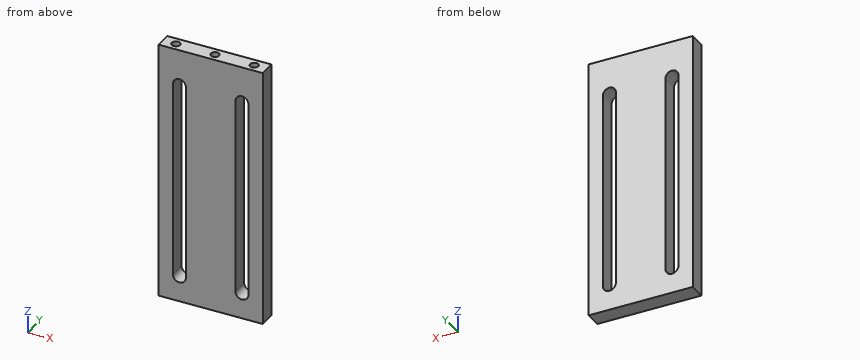
from build123d import *

# Parameters (mm, degrees)
SKETCH1_W           = 20
SKETCH1_H           = 50
BOSS_EXTRUDE1_DEPTH = 3.18
CUT_EXTRUDE1_DEPTH  = 54.94545764
SKETCH3_R           = 0.8
CUT_EXTRUDE2_DEPTH  = 4


with BuildPart() as part:
    # Sketch1 → Boss-Extrude1 (new body)
    with BuildSketch(Plane(origin=(0, 0, 0), x_dir=(1, 0, 0), z_dir=(0, 1, 0))):
        with Locations((10, 25)):
            Rectangle(SKETCH1_W, SKETCH1_H)
    extrude(amount=BOSS_EXTRUDE1_DEPTH)

    # Sketch2 → Cut-Extrude1 (cut, through all)
    with BuildSketch(Plane(origin=(0, 3.18, 0), x_dir=(1, 0, 0), z_dir=(0, 1, 0))):
        with BuildLine():
            Line((2.75, 7), (2.75, 45))
            ThreePointArc((2.75, 45), (4, 46.25), (5.25, 45))
            Line((5.25, 45), (5.25, 7))
            ThreePointArc((5.25, 7), (4, 5.75), (2.75, 7))
        make_face()
    cut_extrude1 = extrude(amount=-CUT_EXTRUDE1_DEPTH, mode=Mode.SUBTRACT)

    # Mirror1: Cut-Extrude1 across plane
    add(cut_extrude1.mirror(Plane(origin=(10, 0, 0), x_dir=(0, 0, 1), z_dir=(1, 0, 0))), mode=Mode.SUBTRACT)

    # Sketch3 → Cut-Extrude2 (cut)
    with BuildSketch(Plane.XY):
        with Locations((10, 1.59)):
            Circle(SKETCH3_R)
        with Locations((2.5, 1.59)):
            Circle(SKETCH3_R)
        with Locations((17.5, 1.59)):
            Circle(SKETCH3_R)
    extrude(amount=-CUT_EXTRUDE2_DEPTH, mode=Mode.SUBTRACT)


solid = part.part
Model file for the job. Use its own axes, mm. Give positions to 0.01 mm unless a question says otherwise; leave off trailing zeros. Order: outer loops, then holes, each group sorted by start corner. A loop starts at its lowest first (then second) coordinate and runs counter-clockwise, first axis right, second up. Notation, with made-up numbers: M -31,-26 L 27,-26 A16 ccw 27,-8 Z; hole C 44,-36 d5. An arc over 180 degrees is marked long. Put each result on its own line as item: value. Start each with the question number.
(1) Pin check, flat tips, straight feed: pin 1 Ø0.5 at (x, y) = (2, 1.5) entering from +Z; pin 2 Ø1 at (y, z) = (1.5, -17) entering from -X. Stop position of each tip, or through.
(2) Band-saw the part on C-C on y = 1.59. Give the cut face in (x, z).
(3) Drill centre lines: L1, parallel to X at y = 1.2, z = -16.5; L2, parallel to Y at x = 10, z = -1.4; L3, parallel to Z at x = 10.5, y = 1.95. Where is each one in solid material? Low to high. Write a range as [from, to].
(4) Band-saw the part on B-B on z = -37.5. Give the cut face in (x, y).
(5) Band-saw the part on A-A on x = 4. Give the cut face in (y, z), then the cut area to 3 significant figures.
(6) Band-saw the part on D-D on x = 10. Give the cut face in (y, z), then the cut area to 3 significant figures.
Results below:
1. pin 1: stops at z = -4
1. pin 2: stops at x = 0
2. outline: M 0,-50 L 20,-50 L 20,0 L 18.3,0 L 18.3,-4 L 16.7,-4 L 16.7,0 L 10.8,0 L 10.8,-4 L 9.2,-4 L 9.2,0 L 3.3,0 L 3.3,-4 L 1.7,-4 L 1.7,0 L 0,0 Z; hole M 2.75,-45 A1.25 ccw 5.25,-45 L 5.25,-7 A1.25 ccw 2.75,-7 Z; hole M 14.75,-45 A1.25 ccw 17.25,-45 L 17.25,-7 A1.25 ccw 14.75,-7 Z
3. L1: x = [0, 2.75], [5.25, 14.75], [17.25, 20]
3. L2: y = [0, 0.79], [2.39, 3.18]
3. L3: z = [-50, -4]
4. outline: M 0,0 L 2.75,0 L 2.75,3.18 L 0,3.18 Z; M 5.25,0 L 14.75,0 L 14.75,3.18 L 5.25,3.18 Z; M 17.25,0 L 20,0 L 20,3.18 L 17.25,3.18 Z
5. outline: M 0,-50 L 3.18,-50 L 3.18,-46.25 L 0,-46.25 Z; M 0,-5.75 L 3.18,-5.75 L 3.18,0 L 0,0 Z
5. area: 30.2 mm2
6. outline: M 0,-50 L 3.18,-50 L 3.18,0 L 2.39,0 L 2.39,-4 L 0.79,-4 L 0.79,0 L 0,0 Z
6. area: 153 mm2
